Input: part model. Units: mm. Frame: model coordinates. A direction names the side the tool comes from. Round coordinates to 2 decimals unless told otherwise and drop trailing zeros. Write each loop counter-clockwise with the first axis right and the second up, starting at its lowest first coordinate (ties: lowest second). Pieces come first, ordered by that corner, then holes. Notation, with made-up numbers: M 85.25,35.5 L 129.25,35.5 A29 cw 129.25,70.5 Z; hole C 17,-1.5 d11. An arc over 180 degrees is marked long. Write each question's results on one line, items separated by ' | '. Start each with the question number.
```python
from build123d import *

# Parameters (mm, degrees)
SKETCH2_W           = 10
SKETCH2_H           = 12
BOSS_EXTRUDE1_DEPTH = 15
FILLET2_R           = 2.5
FILLET3_R           = 2.5
FILLET4_R           = 2.5
FILLET5_R           = 2.5
BOSS_EXTRUDE2_DEPTH = 9
FILLET6_R           = 0.5
SKETCH4_R           = 2
SKETCH4_R_2         = 1.25
BOSS_EXTRUDE4_DEPTH = 0.8
SKETCH5_R           = 1.25
BOSS_EXTRUDE5_DEPTH = 10
CUT_EXTRUDE1_DEPTH  = 9.2
CUT_EXTRUDE2_DEPTH  = 15
BOSS_EXTRUDE7_DEPTH = 20


with BuildPart() as part:
    # Sketch2 → Boss-Extrude1 (new body)
    with BuildSketch(Plane(origin=(0, 0, 0), x_dir=(1, 0, 0), z_dir=(0, 1, 0))):
        with Locations((-5, -6)):
            Rectangle(SKETCH2_W, SKETCH2_H)
    extrude(amount=BOSS_EXTRUDE1_DEPTH)

    # Fillet2
    fillet2_edges = [part.edges().sort_by_distance(p)[0] for p in [
        (0, 7.5, 0),
    ]]
    fillet(fillet2_edges, radius=FILLET2_R)

    # Fillet3
    fillet3_edges = [part.edges().sort_by_distance(p)[0] for p in [
        (-10, 7.5, 0),
    ]]
    fillet(fillet3_edges, radius=FILLET3_R)

    # Fillet4
    fillet4_edges = [part.edges().sort_by_distance(p)[0] for p in [
        (-10, 7.5, 12),
    ]]
    fillet(fillet4_edges, radius=FILLET4_R)

    # Fillet5
    fillet5_edges = [part.edges().sort_by_distance(p)[0] for p in [
        (0, 7.5, 12),
    ]]
    fillet(fillet5_edges, radius=FILLET5_R)

    # Sketch3 → Boss-Extrude2 (add)
    with BuildSketch(Plane.XZ):
        with BuildLine():
            Line((0, 0), (0, 2.5))
            ThreePointArc((0, 2.5), (-0.732233047, 0.732233047), (-2.5, 0))
            Line((-2.5, 0), (0, 0))
        make_face()
        with BuildLine():
            ThreePointArc((-2.5, 0), (-0.732233047, 0.732233047), (0, 2.5))
            Line((0, 2.5), (-5, 6))
            Line((-5, 6), (-10, 2.5))
            ThreePointArc((-10, 2.5), (-9.267766953, 0.732233047), (-7.5, 0))
            Line((-7.5, 0), (-2.5, 0))
        make_face()
        with BuildLine():
            ThreePointArc((-7.5, 0), (-9.267766953, 0.732233047), (-10, 2.5))
            Line((-10, 2.5), (-10, 0))
            Line((-10, 0), (-7.5, 0))
        make_face()
        Polygon((-5, 6), (0, 2.5), (0, 9.5), align=None)
        Polygon((-10, 2.5), (-5, 6), (-10, 9.5), align=None)
        with BuildLine():
            Line((-10, 9.5), (-5, 6))
            Line((-5, 6), (0, 9.5))
            ThreePointArc((0, 9.5), (-0.732233047, 11.267766953), (-2.5, 12))
            Line((-2.5, 12), (-7.5, 12))
            ThreePointArc((-7.5, 12), (-9.267766953, 11.267766953), (-10, 9.5))
        make_face()
        with BuildLine():
            Line((-10, 12), (-10, 9.5))
            ThreePointArc((-10, 9.5), (-9.267766953, 11.267766953), (-7.5, 12))
            Line((-7.5, 12), (-10, 12))
        make_face()
        with BuildLine():
            ThreePointArc((-2.5, 12), (-0.732233047, 11.267766953), (0, 9.5))
            Line((0, 9.5), (0, 12))
            Line((0, 12), (-2.5, 12))
        make_face()
    extrude(amount=BOSS_EXTRUDE2_DEPTH)

    # Fillet6
    fillet6_edges = [part.edges().sort_by_distance(p)[0] for p in [
        (0, -4.5, 12),
        (-10, -4.5, 12),
        (-10, -4.5, 0),
        (0, -4.5, 0),
    ]]
    fillet(fillet6_edges, radius=FILLET6_R)

    # Sketch4 → Boss-Extrude4 (add)
    with BuildSketch(Plane.XZ.offset(9)):
        with Locations((-5, 6)):
            Circle(SKETCH4_R)
        with Locations((-5, 6)):
            Circle(SKETCH4_R_2, mode=Mode.SUBTRACT)
    extrude(amount=BOSS_EXTRUDE4_DEPTH)

    # Sketch5 → Boss-Extrude5 (add)
    with BuildSketch(Plane.XZ.offset(9)):
        with Locations((-5, 6)):
            Circle(SKETCH5_R)
    extrude(amount=BOSS_EXTRUDE5_DEPTH)

    # Sketch6 → Cut-Extrude1 (cut)
    with BuildSketch(Plane.XZ.offset(19)):
        with BuildLine():
            Line((-6, 6.75), (-5, 6.75))
            Line((-5, 6.75), (-4, 6.75))
            ThreePointArc((-4, 6.75), (-5, 7.25), (-6, 6.75))
        make_face()
    extrude(amount=-CUT_EXTRUDE1_DEPTH, mode=Mode.SUBTRACT)

    # Sketch8 → Cut-Extrude2 (cut)
    with BuildSketch(Plane(origin=(0, 15, 0), x_dir=(1, 0, 0), z_dir=(0, 1, 0))):
        with BuildLine():
            Line((-7.5, -12), (-2.5, -12))
            ThreePointArc((-2.5, -12), (-0.732233047, -11.267766953), (0, -9.5))
            Line((0, -9.5), (0, -2.5))
            ThreePointArc((0, -2.5), (-0.732233047, -0.732233047), (-2.5, 0))
            Line((-2.5, 0), (-7.5, 0))
            ThreePointArc((-7.5, 0), (-9.267766953, -0.732233047), (-10, -2.5))
            Line((-10, -2.5), (-10, -9.5))
            ThreePointArc((-10, -9.5), (-9.267766953, -11.267766953), (-7.5, -12))
        make_face()
    extrude(amount=-CUT_EXTRUDE2_DEPTH, mode=Mode.SUBTRACT)

    # Sketch9 → Boss-Extrude7 (add)
    with BuildSketch(Plane(origin=(0, 0, 0), x_dir=(1, 0, 0), z_dir=(0, 1, 0))):
        with BuildLine():
            Line((0, -9.31662479), (0, -2.68337521))
            ThreePointArc((0, -2.68337521), (-5, 0), (-10, -2.68337521))
            Line((-10, -2.68337521), (-10, -9.31662479))
            ThreePointArc((-10, -9.31662479), (-5, -12), (0, -9.31662479))
        make_face()
    extrude(amount=BOSS_EXTRUDE7_DEPTH)


solid = part.part
```
1. Access query for faces 5 (the face through (-1, 0, 11)), 6 (the face through (-9, 0, 11)), 7 (the face through (-2.8, -9, 6.1)), 8 (the face through (-9, 0, 1)), 9 (the face through (-1, 0, 1)). Directions: +Z, -Z, +X, -X, +Y, -Y. A direction counts if a zero-diameter tool reaches every point of the face in a straight line with its end or side. Return the directions, or none.
2. Contact query for flat-ended pins moving along their axis: P1, Ø0.6, axis at x = -5, y = -15, coming from the +Z side; P2, Ø0.8, axis at x = -8.5, z = 0.5, coming from the +Y side; P3, Ø1.5, axis at x = -6, z = 1.5, coming from the -Y side. Output: stop coordinate, or through.
3. Cut plane B-B on x = -9. Output: boundary loops of the cut face in (y, z), and give its area (3 significant figures).
4. Line query: L1, parallel to Y at x = -5.5, z = 7.75; L2, parallel to Y at x = -1.5, z = 5.75; L3, parallel to Z at x = -5.25, y = 14. Output: solid intervals per line, ascending. Write a range as from..to.
5. Cut plane D-D on z = 10. Output: boundary loops of the cut face in (x, y), and give its area (3 significant figures).
6. Cut plane C-C on y = 16.5. Output: boundary loops of the cut face in (x, z).
7. Draft query along X for faces 1 (the face through (-10, 2, 6)), 2 (the face through (-5, -9.8, 7)), 3 (the face through (0, 2, 6)), 4 (the face through (-5, 10, 12)). Return one class per face: +X half, -X half, draft (parallel to the pull), parting line (faces both ways), or undercut.
8. Cut plane A-A on z = 6. Output: boundary loops of the cut face in (x, y).
Answers follow:
1) face 5: +Z, +X, +Y | face 6: +Z, -X, +Y | face 7: -Y | face 8: -Z, -X, +Y | face 9: -Z, +X, +Y
2) P1: stops at z = 6.75 | P2: stops at y = 0 | P3: stops at y = -9
3) outline: M -9,0 L 0,0 L 0,1.53 L 20,1.53 L 20,10.47 L 0,10.47 L 0,12 L -9,12 Z | area: 287 mm2
4) L1: y = -9.8..20 | L2: y = -9..20 | L3: z = 0.01..11.99
5) outline: M -10,-9 L 0,-9 L 0,0 L -0.53,0 L -0.53,20 L -9.47,20 L -9.47,0 L -10,0 Z | area: 269 mm2
6) outline: M -10,2.68 A6 ccw 0,2.68 L 0,9.32 A6 ccw -10,9.32 Z
7) face 1: -X half | face 2: draft | face 3: +X half | face 4: parting line
8) outline: M -10,-9 L -7,-9 L -7,-9.8 L -6.25,-9.8 L -6.25,-19 L -3.75,-19 L -3.75,-9.8 L -3,-9.8 L -3,-9 L 0,-9 L 0,20 L -10,20 Z
